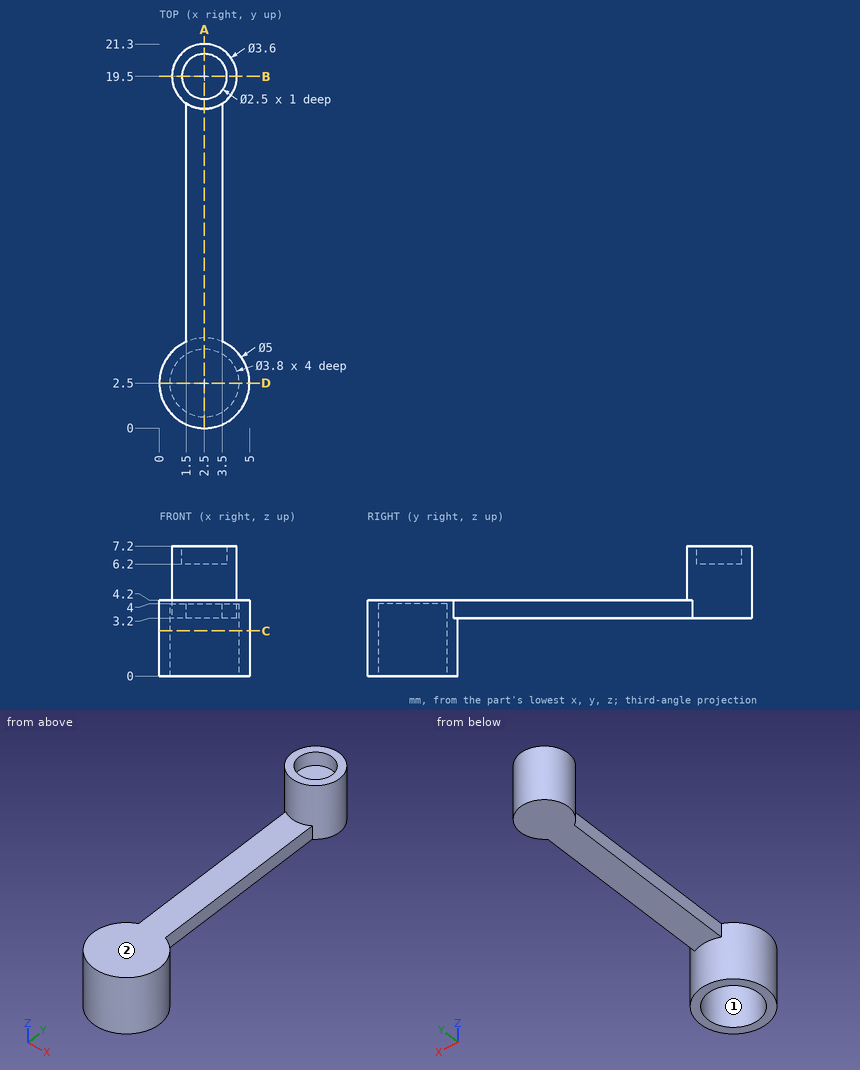
Part print with two shaded views. Sizes in mm from the minimum x, y, z corner. Coordinates: 2 decimals unless noted, no trailing zeros. Write each loop counter-clockwise with the first axis right and the second up, starting at its lowest first coordinate (ties: lowest second). Pieces come first, ordered by that corner, then holes. Notation, with made-up numbers: (14.25, 29) -> (19.25, 29) arc R11 ccw to (19.25, 34) -> close; hole circle Ø7 at (89.25, 2.5). An arc over 180 degrees is marked (long way). Return JSON: item names as keys, results as strings. Group by question number.
Q1. Flat gauge pins, fed straight in: pin 1 (1.5 mm diameter, centred on x = 1, z = 5, fed in from +Y); pin 2 (1.5 mm diameter, centred on x = 3, z = 3.5, fed in from -Y); pin 3 (0.8 mm diameter, centred on x = 2.5, y = 19.5, fed in from +Z); pin 4 (1 mm diameter, centred on x = 2, y = 18.5, fed in from -Z). Where does each tip first touch, or does it go through?
Q2. Pull direction Y, two halves, no side cores. Call the marked faces 1 and 2: released by +Y, released by -Y, zero draft, split by the parting line, or undercut.
Q3. Cut at B-B, the plane y = 19.5. Give the cut face in (x, z).
Q4. Cut at D-D, the plane y = 2.5. Give the cut face in (x, z).
Q5. Cut at A-A, the plane x = 2.5. Give the cut face in (y, z).
Q6. Drill centre lines: line 1 (Y direction, x = 2.4, z = 2.5); line 2 (Y direction, x = 2.5, z = 6.6); line 3 (Z direction, x = 2.85, y = 2.5). Where is each one in solid material? Low to high.
Q7. Cut at C-C, the plane z = 2.5. Give the cut face in (x, y), then the cut area to 3 significant figures.
Returned:
{
 "1": {"pin 1": "stops at y = 21.14", "pin 2": "stops at y = 0", "pin 3": "stops at z = 6.2", "pin 4": "stops at z = 3.2"},
 "2": {"face 1": "undercut", "face 2": "zero draft"},
 "3": {"outline": "(0.7, 3.2) -> (4.3, 3.2) -> (4.3, 7.2) -> (3.75, 7.2) -> (3.75, 6.2) -> (1.25, 6.2) -> (1.25, 7.2) -> (0.7, 7.2) -> close"},
 "4": {"outline": "(0, 0) -> (0.6, 0) -> (0.6, 4) -> (4.4, 4) -> (4.4, 0) -> (5, 0) -> (5, 4.2) -> (0, 4.2) -> close"},
 "5": {"outline": "(0, 0) -> (0.6, 0) -> (0.6, 4) -> (4.4, 4) -> (4.4, 0) -> (5, 0) -> (5, 3.2) -> (21.3, 3.2) -> (21.3, 7.2) -> (20.75, 7.2) -> (20.75, 6.2) -> (18.25, 6.2) -> (18.25, 7.2) -> (17.7, 7.2) -> (17.7, 4.2) -> (0, 4.2) -> close"},
 "6": {"line 1": "y = 0 to 0.6, 4.4 to 5", "line 2": "y = 17.7 to 18.25, 20.75 to 21.3", "line 3": "z = 4 to 4.2"},
 "7": {"outline": "circle Ø5 at (2.5, 2.5); hole circle Ø3.8 at (2.5, 2.5)", "area": "8.29 mm2"}
}
